Job drawing, mm, ordinate dimensions from the low corner. One solid piece. Coordinates: 2 decimals unless noted, no trailing zeros. Loops run counter-clockwise (first coordinate to the right, second up) from the corner with the lowest first, then second, coordinate; pieces in that order, holes last. Notation, with made-up numbers: (52, -23.75) -> (71, -23.75) arc R26 cw to (71, 7.25) -> close; hole circle Ø10 at (64.25, 67). An arc over 180 degrees is marked (long way). Answer as CSV lines item,"result". Start each with the question number.
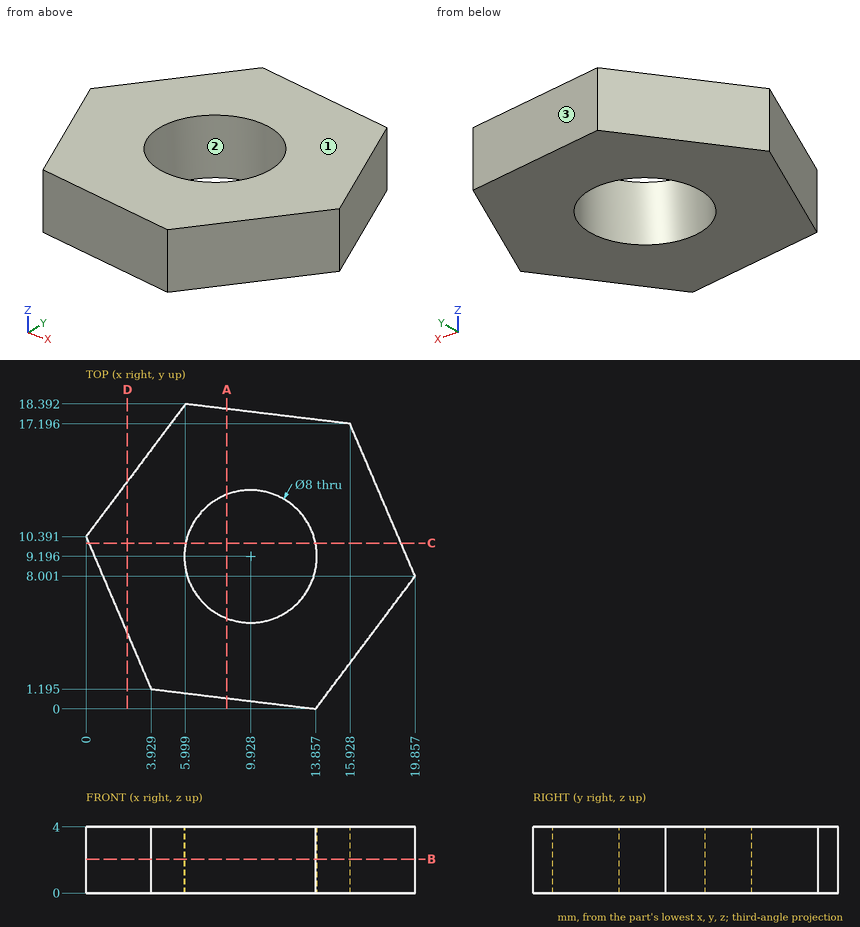
Item 1: Two-plate mould, pull along X, no slides. Class the marked faces 1, 2 and 3: pulls with the +X half, pulls with the -X half, needs draft (parallel to the pull), parting line crosses it, or undercut.
Item 2: Flat gauge pin, fed straight in: pin 1 Ø2 at (x, z) = (15, 0.5) entering from +Y. Where does the tip first touch, or does it go through?
Item 3: Saw through at C-C (y = 10). Write the cut outline in (x, z), plus the area to 3 significant figures.
Item 4: Saw through at A-A (x = 8.5). Write the cut outline in (y, z) (1 decimal), plus the area to 3 significant figures.
Item 5: Saw through at D-D (x = 2.5). Write the cut outline in (y, z) (1 decimal).
Item 6: Wall check: probe 1 along Y at (x, z) = (10, 0.4) (1 decimal); probe 2 along Y at (x, z) = (7, 2.05) (1 decimal); probe 3 along Y at (x, z) = (1.25, 3.75) (1 decimal). Give the ranges that are in metal, low to high.
Item 7: Saw through at B-B (z = 2.05). Write the cut outline in (x, y) (1 decimal).
Geometry check:
1,face 1,"needs draft"
1,face 2,"undercut"
1,face 3,"pulls with the +X half"
2,pin 1,"y = 17.43"
3,outline,"(0.17, 0) -> (6.01, 0) -> (6.01, 4) -> (0.17, 4) -> close; (13.85, 0) -> (19, 0) -> (19, 4) -> (13.85, 4) -> close"
3,area,"44.0 mm2"
4,outline,"(0.6, 0) -> (5.5, 0) -> (5.5, 4) -> (0.6, 4) -> close; (12.9, 0) -> (18.1, 0) -> (18.1, 4) -> (12.9, 4) -> close"
4,area,"39.9 mm2"
5,outline,"(4.5, 0) -> (13.7, 0) -> (13.7, 4) -> (4.5, 4) -> close"
6,probe 1,"0.5 to 5.2, 13.2 to 17.9"
6,probe 2,"0.8 to 6.5, 11.9 to 18.3"
6,probe 3,"7.5 to 12.1"
7,outline,"(0, 10.4) -> (3.9, 1.2) -> (13.9, 0) -> (19.9, 8) -> (15.9, 17.2) -> (6, 18.4) -> close; hole circle Ø8 at (9.9, 9.2)"
